from build123d import *

# Parameters (mm, degrees)
BOX247_W                  = 0.5
BOX247_H                  = 1
BOX247_DEPTH              = 15
BOX247_ROLL_ANGLE         = 46
BOX248_W                  = 0.5
BOX248_H                  = 1
BOX248_DEPTH              = 15
BOX248_ROLL_ANGLE         = -46
BOX246_W                  = 0.5
BOX246_H                  = 1
BOX246_DEPTH              = 11
FUSION025_PLACEMENT_ANGLE = -51.1


with BuildPart() as cubo247:
    # Box247 → Box247 (new body)
    with BuildSketch(Plane.XY):
        with Locations((0.25, 0.5)):
            Rectangle(BOX247_W, BOX247_H)
    extrude(amount=BOX247_DEPTH)


with BuildPart() as cubo247_1:
    # Box247 roll: moved
    add(cubo247.part.rotate(Axis((0, 0, 0), (1, 0, 0)), BOX247_ROLL_ANGLE))


with BuildPart() as cubo247_2:
    # Box247 placement: moved
    add(cubo247_1.part.moved(Location((0, 11, 0.5))))


with BuildPart() as cubo248:
    # Box248 → Box248 (new body)
    with BuildSketch(Plane.XY):
        with Locations((0.25, 0.5)):
            Rectangle(BOX248_W, BOX248_H)
    extrude(amount=BOX248_DEPTH)


with BuildPart() as cubo248_1:
    # Box248 roll: moved
    add(cubo248.part.rotate(Axis((0, 0, 0), (1, 0, 0)), BOX248_ROLL_ANGLE))


with BuildPart() as cubo248_2:
    # Box248 placement: moved
    add(cubo248_1.part.moved(Location((0, 0.4, 1.1))))


with BuildPart() as fusion025:
    # Box246 → Box246 (new body)
    with BuildSketch(Plane.XY.offset(0.5)):
        with Locations((0.25, 0.5)):
            Rectangle(BOX246_W, BOX246_H)
    extrude(amount=BOX246_DEPTH)

    # Fusion025: union Cubo247, Cubo248
    add(cubo247_2.part)
    add(cubo248_2.part)


with BuildPart() as fusion025_1:
    # Fusion025 placement: moved
    add(fusion025.part.moved(Location((-155.2, 175.6, 0))).rotate(Axis((-155.2, 175.6, 0), (0, 0, 1)), FUSION025_PLACEMENT_ANGLE))


solid = fusion025_1.part
For this review, take the finished solid that the model builds, in its own axes (mm). A direction names the side the tool comes from. Round coordinates to 2 decimals unless told otherwise and drop trailing zeros. Order: outer loops, then holes, each group sorted by start corner. A loop starts at its lowest first (then second) coordinate and runs counter-clockwise, first axis right, second up. Notation, with made-up numbers: (87.5, 49.5) -> (122.5, 49.5) arc R26 cw to (122.5, 78.5) -> close; hole circle Ø8 at (65, 23.5). An arc over 180 degrees is marked (long way). Write item = value, one per line. Start each with the question number.
1) Take a section at B-B on y = 177.25. State the section outline as (x, z) points.
2) Tool access review of faces 1 (the face through (-154.7, 175.7, 0.5)), 2 (the face through (-146.062, 182.656, 11.155)), 3 (the face through (-147.791, 181.262, 8.325)): name each direction out of +Z, -Z, +X, -X, +Y, -Y from which nothing blocks a thin tool from reaching the whole face with its end or side.
3) The part is to be moulded in two halves that separate along Z. For faces 4 (the face through (-154.7, 175.7, 11.5)), 5 (the face through (-150.88, 179.086, 6.001)), 6 (the face through (-152.583, 177.395, 3.769)), 7 (the face through (-146.21, 182.537, 0.865)), say which applies: +Z half, -Z half, draft (parallel to the pull), parting line (faces both ways), or undercut.
4) Take a section at C-C on z = 3. State the section outline as (x, y) points.
5) Insertion check: pin 1 (3 mm diameter, centred on y = 179.5, z = 7, fed in from -X); pin 2 (1.5 mm diameter, centred on x = -152.5, z = 6.5, fed in from -Y); pin 3 (1.5 mm diameter, centred on x = -152.5, z = 7, fed in from +Y); pin 4 (1.1 mm diameter, centred on x = -155, y = 175.5, fed in from -Z). Each pin has a flat end and moves straight along its axis. Give the tip position at first contact, or say it passes through.
6) To check wall thickness, follow line 1 (Z direction, x = -154, y = 176.5); line 2 (X direction, y = 176, z = 10.75); line 3 (Y direction, x = -154.5, z = 5.25). State the ranges of each line that lie inside material, in increasing order. Write a range as from..to.
7) Take a section at D-D on y = 178.75. State the section outline as (x, z) points.
8) Take a section at A-A on z = 11.25. State the section outline as (x, y) points.
Verdict:
q1.outline = (-153.16, 1.86) -> (-152.36, 2.46) -> (-152.36, 3.85) -> (-153.16, 3.25) -> close; (-153.16, 8.59) -> (-152.36, 7.99) -> (-152.36, 9.38) -> (-153.16, 9.98) -> close
q2.face_1 = -Z, -X, -Y
q2.face_2 = +Z, +X, +Y
q2.face_3 = +X, +Y
q3.face_4 = +Z half
q3.face_5 = draft
q3.face_6 = undercut
q3.face_7 = -Z half
q4.outline = (-155.2, 175.6) -> (-154.89, 175.21) -> (-154.11, 175.84) -> (-154.42, 176.23) -> close; (-153.36, 177.09) -> (-153.04, 176.7) -> (-151.92, 177.6) -> (-152.24, 177.99) -> close; (-148.65, 180.88) -> (-148.34, 180.49) -> (-147.22, 181.4) -> (-147.53, 181.79) -> close
q5.pin_1 = -152.17
q5.pin_2 = through
q5.pin_3 = 178.38
q5.pin_4 = 0.5
q6.line_1 = 0.77..2.16, 9.67..11.07
q6.line_2 = -154.7..-153.91
q6.line_3 = 175.52..176.16
q7.outline = (-151.3, 4.17) -> (-150.5, 4.77) -> (-150.5, 7.07) -> (-151.3, 7.67) -> (-151.3, 6.28) -> (-150.82, 5.92) -> (-151.3, 5.56) -> close
q8.outline = (-155.2, 175.6) -> (-154.89, 175.21) -> (-153.87, 176.03) -> (-154.18, 176.42) -> close; (-146.71, 182.45) -> (-146.39, 182.06) -> (-145.97, 182.4) -> (-146.29, 182.79) -> close
